Print and shaded views of the part. All mm, measured from the part's lowest x, y and z. A direction names the side the tool comes from. Give positions to 0.01 mm unless a question says otherwise; leave off trailing zeros. Loops run counter-clockwise (first coordinate to the right, second up) from the corner with the lowest first, then second, coordinate; pieces in that order, holes last. Notation, with made-up numbers: M 49.5,69.25 L 100.5,69.25 A18 cw 100.5,96.25 Z; hole C 84,41 d11. An arc over 180 degrees is marked long. Answer as CSV lines item,"result".
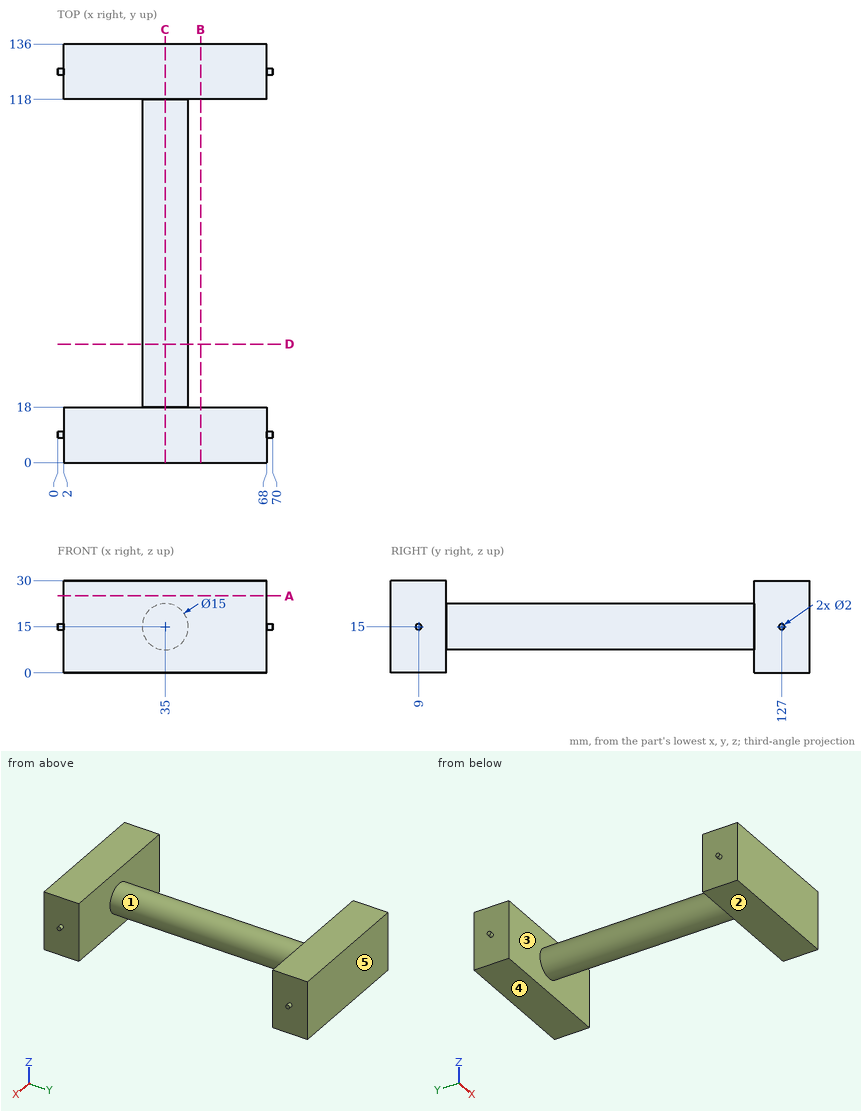
Q1. Mould opens along Y. For the marked faces 3, 4 and 5 say: released by +Y, released by -Y, zero draft, split by the parting line, or undercut.
Solution:
face 3,"undercut"
face 4,"zero draft"
face 5,"released by +Y"
Q2. Which spindle directions (+Z, -Z, +X, -X, +Y, -Y) get a long thin tool onto all of the face, cutting with end or side? Do the marked faces 1 and 2. Say none if no direction does.
Solution:
face 1,"none"
face 2,"-Z, +X, -X, +Y, -Y"
Q3. Cut at D-D (y = 38.5). Write the cut outline in (x, z), and give its area (3 significant figures).
Solution:
outline,"C 35,15 d15"
area,"177 mm²"
Q4. Cut at C-C (x = 35). Write the cut outline in (y, z).
Solution:
outline,"M 0,0 L 18,0 L 18,7.5 L 118,7.5 L 118,0 L 136,0 L 136,30 L 118,30 L 118,22.5 L 18,22.5 L 18,30 L 0,30 Z"
Q5. Cut at B-B (x = 46.5). Write the cut outline in (y, z).
Solution:
outline,"M 0,0 L 18,0 L 18,30 L 0,30 Z; M 118,0 L 136,0 L 136,30 L 118,30 Z"
Q6. Wall check: line 1 (Y direction, x = 20.5, z = 15.5); line 2 (X direction, y = 19.5, z = 14.5); line 3 (X direction, y = 13, z = 16.5). Give the ranges that are in metal, low to high. Write a range as [from, to].
Solution:
line 1,"y = [0, 18], [118, 136]"
line 2,"x = [27.52, 42.48]"
line 3,"x = [2, 68]"
Q7. Cut at A-A (z = 25). Write the cut outline in (x, y), and give its area (3 significant figures).
Solution:
outline,"M 2,0 L 68,0 L 68,18 L 2,18 Z; M 2,118 L 68,118 L 68,136 L 2,136 Z"
area,"2,380 mm²"
Q8. Pin check, flat tips, straight feed: P1, Ø9, axis at y = 125.5, z = 9, coming from the -X side; P2, Ø8, axis at x = 45.5, y = 28, coming from the +Z side; P3, Ø3, axis at y = 71, z = 13.5, coming from the +X side. Stop position of each tip, or through.
Solution:
P1,"stops at x = 2"
P2,"stops at z = 18.74"
P3,"stops at x = 42.5"
